```python
from build123d import *

# Parameters (mm, degrees)
SKETCH1_W           = 130
SKETCH1_H           = 90
BOSS_EXTRUDE1_DEPTH = 37.58
SKETCH2_W           = 10
SKETCH2_H           = 100
BOSS_EXTRUDE2_DEPTH = 5
SKETCH3_W           = 85
SKETCH3_H           = 10
BOSS_EXTRUDE3_DEPTH = 5


with BuildPart() as part:
    # Sketch1 → Boss-Extrude1 (new body)
    with BuildSketch(Plane(origin=(0, 0, 0), x_dir=(1, 0, 0), z_dir=(0, 1, 0))):
        with Locations((65, -45)):
            Rectangle(SKETCH1_W, SKETCH1_H)
    extrude(amount=BOSS_EXTRUDE1_DEPTH)

    # Sketch2 → Boss-Extrude2 (add)
    with BuildSketch(Plane.ZY):
        with Locations((45, 50)):
            Rectangle(SKETCH2_W, SKETCH2_H)
    extrude(amount=BOSS_EXTRUDE2_DEPTH)

    # Sketch3 → Boss-Extrude3 (add)
    with BuildSketch(Plane(origin=(0, 100, 0), x_dir=(1, 0, 0), z_dir=(0, 1, 0))):
        with Locations((37.5, -45)):
            Rectangle(SKETCH3_W, SKETCH3_H)
    extrude(amount=BOSS_EXTRUDE3_DEPTH)


solid = part.part
```
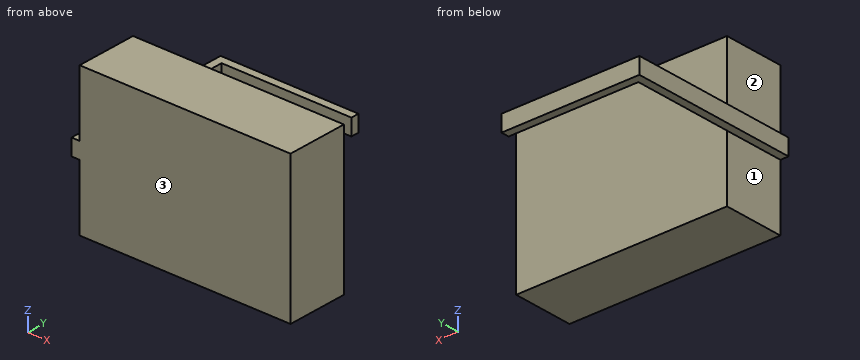
Here's how the part is built. I have some questions about the finished solid (model axes, mm). Face numbers are marked on the shaded views. A direction names the side the tool comes from. Give positions to 0.01 mm unless a question says otherwise; leave off trailing zeros. Loops run counter-clockwise (first coordinate to the right, second up) from the corner with the lowest first, then second, coordinate; pieces in that order, holes last. Notation, with made-up numbers: M 67.25,31.5 L 74.25,31.5 A28 cw 74.25,49.5 Z; hole C -4,20 d7. An arc over 180 degrees is marked long. Put each result on its own line as item: value. Start each with the question number.
(1) For the marked faces 1, 2 and 3, which set-ups out of +Z, -Z, +X, -X, +Y, -Y let a thin tool reach every point of the face, with its end or its side?
(2) I need wall thicknesses on line 1 along X through (y, z) = (7, 15); line 2 along Y through (x, z) = (46, 22). Which ranges of each line are inside material? Lowest first, please. Write a range as [from, to].
(3) I want a section at A-A on x = 59.5. Please give me the cut outline in (y, z), then the cut area to 3 significant figures.
(4) Will these pins go through, and if not, where does the flat tip stop? pin 1 Ø3 at (y, z) = (66.5, 43.5) entering from +X; pin 2 Ø1.5 at (y, z) = (102.5, 46.5) entering from +X.
(5) I want a section at B-B on z = 45.5. Please give me the cut outline in (x, y), then the cut area to 3 significant figures.
(6) I want a section at C-C on y = 9.5. Please give me the cut outline in (x, z).
(7) I want a section at D-D on x = 93.5. Please give me the cut outline in (y, z).
Answer block:
1. face 1: -Z, -X, +Y, -Y
1. face 2: +Z, -X, +Y, -Y
1. face 3: +Z, -Z, +X, -X, -Y
2. line 1: [0, 130]
2. line 2: [0, 37.58]
3. outline: M 0,0 L 37.58,0 L 37.58,90 L 0,90 Z; M 100,40 L 105,40 L 105,50 L 100,50 Z
3. area: 3,430 mm^2
4. pin 1: x = 0
4. pin 2: x = 80
5. outline: M -5,0 L 130,0 L 130,37.58 L 0,37.58 L 0,100 L 80,100 L 80,105 L -5,105 Z
5. area: 5,810 mm^2
6. outline: M -5,40 L 0,40 L 0,0 L 130,0 L 130,90 L 0,90 L 0,50 L -5,50 Z
7. outline: M 0,0 L 37.58,0 L 37.58,90 L 0,90 Z
